The listing builds one solid part. Answer for the finished solid, in the listing's coordinates (mm). A direction names the side the tool comes from. Round coordinates to 2 decimals unless told otherwise and drop trailing zeros. Order: outer loops, then holes, each group sorted by start corner. A loop starts at its lowest first (then second) coordinate and runs counter-clockwise, first axis right, second up. Notation, with made-up numbers: (57.25, 86.5) - (102.25, 86.5) arc R35 ccw to (102.25, 120.5) - close; hole circle Ø8 at (-36.5, -8.5). An arc over 180 degrees is marked (long way). Write item = value, one per line.
from build123d import *

# Parameters (mm, degrees)
SKETCH_1_R          = 65.5
SKETCH_1_R_2        = 35.5
SKETCH_1_R_3        = 5.1
EXTRUDE_1_DEPTH     = 6
SKETCH_2_R          = 65.5
SKETCH_2_R_2        = 60.5
CUT_EXTRUDE_1_DEPTH = 2


with BuildPart() as part:
    # Эскиз1 → Бобышка-Вытянуть1 (new, symmetric)
    with BuildSketch(Plane(origin=(0, 0, 0), x_dir=(0, 0, -1), z_dir=(1, 0, 0))):
        Circle(SKETCH_1_R)
        Circle(SKETCH_1_R_2, mode=Mode.SUBTRACT)
        with Locations((0, 50.5)):
            Circle(SKETCH_1_R_3, mode=Mode.SUBTRACT)
        with Locations((35.70889245, 35.70889245)):
            Circle(SKETCH_1_R_3, mode=Mode.SUBTRACT)
        with Locations((50.5, 0)):
            Circle(SKETCH_1_R_3, mode=Mode.SUBTRACT)
        with Locations((35.70889245, -35.70889245)):
            Circle(SKETCH_1_R_3, mode=Mode.SUBTRACT)
        with Locations((0, -50.5)):
            Circle(SKETCH_1_R_3, mode=Mode.SUBTRACT)
        with Locations((-35.70889245, -35.70889245)):
            Circle(SKETCH_1_R_3, mode=Mode.SUBTRACT)
        with Locations((-50.5, 0)):
            Circle(SKETCH_1_R_3, mode=Mode.SUBTRACT)
        with Locations((-35.70889245, 35.70889245)):
            Circle(SKETCH_1_R_3, mode=Mode.SUBTRACT)
    extrude(amount=EXTRUDE_1_DEPTH, both=True)

    # Эскиз2 → Вырез-Вытянуть1 (cut)
    with BuildSketch(Plane(origin=(6, 0, 0), x_dir=(0, 0, -1), z_dir=(1, 0, 0))):
        Circle(SKETCH_2_R)
        Circle(SKETCH_2_R_2, mode=Mode.SUBTRACT)
    extrude(amount=-CUT_EXTRUDE_1_DEPTH, mode=Mode.SUBTRACT)


solid = part.part
Q1. Find the intervals of material crossed by line 1 (Y direction, x = 0, z = 0); line 2 (Y direction, x = -2, z = 36); line 3 (Z direction, x = -5, y = -1.5), in increasing order. Write a range as from..to.
Model answer:
line_1 = -65.5..-55.6, -45.4..-35.5, 35.5..45.4, 55.6..65.5
line_2 = -54.72..-40.8, -30.62..30.62, 40.8..54.72
line_3 = -65.48..-55.37, -45.63..-35.47, 35.47..45.63, 55.37..65.48
Q2. Section B-B on z = 29 is taken. Determine the outline of the cut face in (x, y).
Model answer:
outline = (-6, -58.73) - (4, -58.73) - (4, -53.1) - (6, -53.1) - (6, -20.48) - (-6, -20.48) - close; (-6, 20.48) - (6, 20.48) - (6, 53.1) - (4, 53.1) - (4, 58.73) - (-6, 58.73) - close
Q3. For faces 4 (the face through (-0.084, -35.485, -30.614)), 5 (the face through (4, -58, -19)), determine the directions among +Z, -Z, +X, -X, +Y, -Y from which every point of the face is accessible in a straight line to the end or side of a thin tool.
Model answer:
face_4 = +X, -X
face_5 = +X
Q4. Flat-ended cylindrical pins translate along their axes: P1, Ø16.5, axis at y = 50.5, z = 0, coming from the +X side; P2, Ø5, axis at x = 1.5, y = -5, coming from the -Z side; P3, Ø5, axis at x = -3.5, y = 25, coming from the -Z side. Find the tip coordinate at first contact, or state that the pin passes through.
Model answer:
P1 = 6
P2 = -65.45
P3 = -61.51
Q5. Determine the mould class of faces 1 (the face through (-6, -28, -28)), 2 (the face through (5.01, -59.06, 13.12)), 3 (the face through (-0.084, -34.656, 7.696)) for opening direction Z: released by +Z, released by -Z, zero draft, split by the parting line, or undercut.
Model answer:
face_1 = zero draft
face_2 = split by the parting line
face_3 = undercut
Q6. Section D-D on x = 0 is taken. Count the separate pieces of the cut face and the enclosed holes in it, then the cut area to 3 significant figures.
Model answer:
separate_pieces = 1
enclosed_holes = 9
area = 8,870 mm^2
Q7. Section C-C on y = 26.5 is taken. Determine the outline of the cut face in (x, z), then the cut area to 3 significant figures.
Model answer:
outline = (-6, -59.9) - (4, -59.9) - (4, -54.39) - (6, -54.39) - (6, -23.62) - (-6, -23.62) - close; (-6, 23.62) - (6, 23.62) - (6, 54.39) - (4, 54.39) - (4, 59.9) - (-6, 59.9) - close
area = 849 mm^2
Q8. Section A-A on y = 0 is taken. Determine the outline of the cut face in (x, z), then the cut area to 3 significant figures.
Model answer:
outline = (-6, -65.5) - (4, -65.5) - (4, -60.5) - (6, -60.5) - (6, -55.6) - (-6, -55.6) - close; (-6, -45.4) - (6, -45.4) - (6, -35.5) - (-6, -35.5) - close; (-6, 35.5) - (6, 35.5) - (6, 45.4) - (-6, 45.4) - close; (-6, 55.6) - (6, 55.6) - (6, 60.5) - (4, 60.5) - (4, 65.5) - (-6, 65.5) - close
area = 455 mm^2
